Autodesk Inventor part; units mm, degrees
ref_plane "YZ Plane" through (0, 0, 0) normal (1, 0, 0) x (0, 1, 0)
ref_plane "XZ Plane" through (0, 0, 0) normal (0, 1, 0) x (-1, 0, 0)
ref_plane "XY Plane" through (0, 0, 0) normal (0, 0, 1) x (1, 0, 0)
sketch "Sketch1" plane through (0, 0, 0) normal (0, 0, 1) x (1, 0, 0)
  circle A0 centre (10.765, 51.2851) radius 2.1844
  circle A1 centre (31.5233, 19.3366) radius 2.1844
  circle A2 centre (86.9588, 50.3069) radius 2.1844
  circle A3 centre (-3.0738, 72.5841) radius 2.1844
  circle A4 centre (-27.3318, 51.7742) radius 2.1844
  circle A5 centre (-26.0367, 13.3556) radius 2.1844
  arc A6 (30.2901, 14.7365) -> (33.8461, 15.1789) centre (31.5233, 19.3366) ccw
  arc A7 (89.2815, 46.1492) -> (87.0199, 55.069) centre (86.9588, 50.3069) ccw
  arc A8 (-1.1199, 76.9273) -> (-6.1747, 76.1988) centre (-3.0738, 72.5841) ccw
  arc A9 (-30.4327, 55.3889) -> (-32.0916, 51.6137) centre (-27.3318, 51.7742) ccw
  arc A10 (-30.7965, 13.1952) -> (-23.8841, 9.1074) centre (-26.0367, 13.3556) ccw
  line L0 (30.721, 29.3126) -> (6.3194, 66.8684)
  line L1 (-6.1747, 76.1988) -> (-30.4327, 55.3889)
  line L2 (-32.0916, 51.6137) -> (-30.7965, 13.1952)
  line L3 (33.8461, 15.1789) -> (89.2815, 46.1492)
  line L4 (-4.1028, 65.4266) -> (-16.8864, 54.4601)
  line L5 (9.1377, 45.0485) -> (-15.7743, 19.373)
  line L6 (3.2606, 48.1101) -> (-21.58, 22.5083)
  arc A11 (-1.1199, 76.9273) -> (87.2556, 55.0601) centre (103.0888, 308.5662) ccw
  arc A12 (30.2901, 14.7365) -> (-23.8841, 9.1074) centre (10.5583, -58.8644) ccw
  line L7 (3.0226, 54.4601) -> (-16.8864, 54.4601)
  line L8 (3.2606, 48.1101) -> (-22.4431, 48.1101)
  line L9 (75.984, 49.6309) -> (36.8851, 27.7874)
  arc A13 (23.7023, 22.6325) -> (-15.7743, 19.373) centre (10.5583, -58.8644) ccw
  line L10 (-21.58, 22.5083) -> (-22.4431, 48.1101)
  line L11 (23.7023, 22.6325) -> (9.1377, 45.0485)
  line L12 (3.0226, 54.4601) -> (-4.1028, 65.4266)
  line L13 (10.765, 51.2851) -> (-26.0367, 13.3556) construction
  line L14 (31.5233, 19.3366) -> (42.0802, 62.0019) construction
  line L15 (36.8851, 27.7874) -> (43.6417, 55.0939)
  line L16 (30.721, 29.3126) -> (37.4775, 56.6192)
  arc A14 (6.3194, 66.8684) -> (37.4775, 56.6192) centre (103.0888, 308.5662) ccw
  arc A15 (43.6417, 55.0939) -> (75.984, 49.6309) centre (103.0888, 308.5662) ccw
  point P0 (0, 0)
  dimension "d0" = 9.525
  dimension "d1" = 9.525
  dimension "d2" = 9.525
  dimension "d3" = 9.525
  dimension "d5" = 9.525
  dimension "d7" = 254
  dimension "d8" = 76.2
  dimension "d11" = 6.35
  dimension "d12" = 3.175
  dimension "d18" = 3.175
  dimension "d19" = 3.175
  dimension "d20" = 3.175
  dimension "d21" = 3.175
  dimension "d24" = 6.35
extrude "Extrusion1" add sketch "Sketch1" along normal blind 6.35
fillet "Fillet1" radius 2.54 15 edges at (-15.7743, 19.373, 3.175) (9.1377, 45.0485, 3.175) (-4.1028, 65.4266, 3.175) (6.3194, 66.8684, 3.175) (3.2606, 48.1101, 3.175) (3.0226, 54.4601, 3.175) (-22.4431, 48.1101, 3.175) (-21.58, 22.5083, 3.175) (-16.8864, 54.4601, 3.175) (23.7023, 22.6325, 3.175) (75.984, 49.6309, 3.175) (43.6417, 55.0939, 3.175) (37.4775, 56.6192, 3.175) (30.721, 29.3126, 3.175) (36.8851, 27.7874, 3.175)
properties part number "centralbrace" material "Acetal Resin, White"
CAD build for the part. Positions are in the model's coordinates, mm. A direction names the side the tool comes from. Round coordinates to 2 decimals unless told otherwise and drop trailing zeros. Order: outer loops, then holes, each group sorted by start corner. A loop starts at its lowest first (then second) coordinate and runs counter-clockwise, first axis right, second up. Notation, with made-up numbers: (-36, 86.5) - (-8, 86.5) arc R22 ccw to (-8, 116.5) - close; hole circle Ø10 at (40.5, -27). An arc over 180 degrees is marked (long way). Answer in a Markdown table with one row per item. Add a question column.
(1) Drop flat-ended pins along their axis: pin 1 Ø3 at (x, z) = (13.5, 2.5) entering from -Y; pin 2 Ø3 at (x, z) = (-7, 3.5) entering from -Y; pin 3 Ø3 at (y, z) = (47.5, 5) entering from +X. Give the stop position or say it passes through.
(2) Band-saw the part on A-A on x = 51.5. List the corners of the cut face in (y, z).
(3) Band-saw the part on D-D on z = 5. Count the separate pieces of the cut face and the enclosed holes in it, and give its area (3 significant figures).
(4) Band-saw the part on B-B on y = 39. List the corners of the cut face in (x, z), and give its area (3 significant figures).
(5) 3-axis set-ups, long thin cutter, end or side, ignore diameter. For faces 4 (the face through (2.295, 16.886, 3.131)), 5 (the face through (-0.388, 46.521, 3.219)): which of +Z, -Z, +X, -X, +Y, -Y reach the whole face in a straight line?
(6) Band-saw the part on C-C on x = -14.5. List the corners of the cut face in (y, z).
(7) Mould opens along X. For faces 1 (the face through (-1.07, 34.53, 3.13)), 2 (the face through (-28.4, 9.22, 3.13)), 3 (the face through (15, 43, 0)) say: +X half, -X half, draft (parallel to the pull), parting line (faces both ways), or undercut.
(8) Probe L1, parallel to X at y = 33.5, z = 4.25; L2, parallel to Y at x = -3, z = 5.75; L3, parallel to Y at x = 20, z = 1.5. List the from-to ranges inside material, lowest first. Write a range as [from, to].
Data:
| question | item | result |
|---|---|---|
| 1 | pin 1 | stops at y = 17.21 |
| 1 | pin 2 | stops at y = 14.91 |
| 1 | pin 3 | stops at x = 91.54 |
| 2 | outline | (25.04, 0) - (35.95, 0) - (35.95, 6.35) - (25.04, 6.35) - close; (53.38, 0) - (59.86, 0) - (59.86, 6.35) - (53.38, 6.35) - close |
| 3 | separate pieces | 1 |
| 3 | enclosed holes | 11 |
| 3 | area | 3,360 mm^2 |
| 4 | outline | (-31.67, 0) - (-22.14, 0) - (-22.14, 6.35) - (-31.67, 6.35) - close; (-5.58, 0) - (3.27, 0) - (3.27, 6.35) - (-5.58, 6.35) - close; (13.07, 0) - (24.43, 0) - (24.43, 6.35) - (13.07, 6.35) - close; (33.12, 0) - (39.66, 0) - (39.66, 6.35) - (33.12, 6.35) - close; (56.96, 0) - (76.48, 0) - (76.48, 6.35) - (56.96, 6.35) - close |
| 4 | area | 354 mm^2 |
| 5 | face 4 | +Z, -Z, -Y |
| 5 | face 5 | +Z, -Z |
| 6 | outline | (13.1, 0) - (29.81, 0) - (29.81, 6.35) - (13.1, 6.35) - close; (48.11, 0) - (69.06, 0) - (69.06, 6.35) - (48.11, 6.35) - close |
| 7 | face 1 | undercut |
| 7 | face 2 | parting line |
| 7 | face 3 | draft |
| 8 | L1 | x = [-31.48, -21.95], [-10.92, -2.07], [16.64, 28.24], [31.08, 38.3], [47.11, 66.64] |
| 8 | L2 | y = [16.12, 22.56], [32.54, 41.66], [48.11, 54.46], [63.54, 70.4], [74.77, 77.35] |
| 8 | L3 | y = [16.75, 23.74], [28.33, 45.81], [61.83, 68.54] |
